Can you work these out from the model? Positions are in its coordinate system, mm. A direction names the side the tool comes from. Give positions to 0.01 mm unless a question says otherwise; leave off trailing zeros. Loops run counter-clockwise (first coordinate to the right, second up) from the corner with the lowest first, then second, coordinate; pieces in that order, holes last. Notation, with made-up numbers: (54, 58.25) - (94, 58.25) arc R29 cw to (94, 91.25) - close; hole circle Ø8 at (76, -27). An arc over 180 degrees is marked (long way). Write item = value, one per line.
from build123d import *

# Parameters (mm, degrees)
F0_R     = 6.75
F1_DEPTH = 8
F3_DEPTH = 8.001


with BuildPart() as f1:
    # F0 (on Right) → F1 (new body)
    with BuildSketch(Plane.YZ):
        Circle(F0_R)
    extrude(amount=F1_DEPTH)

    # F2 (on face) → F3 (cut, through all)
    with BuildSketch(Plane.YZ.offset(8)):
        with BuildLine():
            ThreePointArc((-1.426585, 0.463525), (-1.256585, 0.819143), (-0.999817, 1.118198))
            Line((-0.999817, 1.118198), (-3.928516, 3.849254))
            ThreePointArc((-3.928516, 3.849254), (-4.704102, 2.849811), (-5.230811, 1.699593))
            Line((-5.230811, 1.699593), (-1.426585, 0.463525))
        make_face()
        with BuildLine():
            Line((-3.232819, -4.449593), (-0.881678, -1.213525))
            ThreePointArc((-0.881678, -1.213525), (-1.167357, -0.941954), (-1.37243, -0.60534))
            Line((-1.37243, -0.60534), (-4.874837, -2.546756))
            ThreePointArc((-4.874837, -2.546756), (-4.163979, -3.593227), (-3.232819, -4.449593))
        make_face()
        with BuildLine():
            ThreePointArc((0, 1.5), (0.390745, 1.448212), (0.754509, 1.296424))
            Line((0.754509, 1.296424), (2.44688, 4.925726))
            ThreePointArc((2.44688, 4.925726), (1.256683, 5.354507), (0, 5.5))
            Line((0, 5.5), (0, 1.5))
        make_face()
        with BuildLine():
            Line((3.232819, -4.449593), (0.881678, -1.213525))
            ThreePointArc((0.881678, -1.213525), (0.535118, -1.401302), (0.151609, -1.492319))
            Line((0.151609, -1.492319), (0.915702, -5.423236))
            ThreePointArc((0.915702, -5.423236), (2.130622, -5.070547), (3.232819, -4.449593))
        make_face()
        with BuildLine():
            ThreePointArc((1.426585, 0.463525), (1.481533, 0.234652), (1.5, 0))
            ThreePointArc((1.5, 0), (1.491508, -0.159384), (1.466129, -0.316964))
            Line((1.466129, -0.316964), (5.440771, -0.804988))
            ThreePointArc((5.440771, -0.804988), (5.485173, -0.403582), (5.5, 0))
            ThreePointArc((5.5, 0), (5.432286, 0.86039), (5.230811, 1.699593))
            Line((5.230811, 1.699593), (1.426585, 0.463525))
        make_face()
    extrude(amount=-F3_DEPTH, mode=Mode.SUBTRACT)


solid = f1.part
Q1. Imagine slicing it at D-D, the plane y = 6.25. Write out the boundary of the cut face in (x, z).
Output:
outline = (0, -2.55) - (8, -2.55) - (8, 2.55) - (0, 2.55) - close
Q2. Which directions (+Z, -Z, +X, -X, +Y, -Y) give clear straight access to the entire face, cutting with the end or side of a thin tool? Please do faces 4 (the flat face through (8, 0, 0)), 5 (the flat face through (4.056, -3.099, -1.562)).
Output:
face_4 = +Z, -Z, +X, +Y, -Y
face_5 = +X, -X
Q3. For pin 1 (2 mm diameter, centred on x = 4, z = -4, fed in from +Y), with a flat end and sliding along its axis, tell me the tip position at first contact or that it passes through.
Output:
pin_1 = 6.05
Q4. We'd pull the mould along Y, two halves only. Please class faces 1 (the flat face through (4.06, -3.36, 1.09)), 2 (the flat face through (0, 0, 0)), 3 (the cylindrical face through (3.94, -1.46, -6.59)): released by +Y, released by -Y, zero draft, split by the parting line, or undercut.
Output:
face_1 = undercut
face_2 = zero draft
face_3 = split by the parting line
Q5. Imagine slicing it at B-B, the plane z = 2.75. Write out the boundary of the cut face in (x, y).
Output:
outline = (0, -6.16) - (8, -6.16) - (8, -4.76) - (0, -4.76) - close; (0, -2.75) - (8, -2.75) - (8, 0) - (0, 0) - close; (0, 1.43) - (8, 1.43) - (8, 6.16) - (0, 6.16) - close
Q6. Imagine slicing it at C-C, the plane y = 2. Write out the boundary of the cut face in (x, z).
Output:
outline = (0, -6.45) - (8, -6.45) - (8, -5.12) - (0, -5.12) - close; (0, -2.75) - (8, -2.75) - (8, -0.38) - (0, -0.38) - close; (0, 0.65) - (8, 0.65) - (8, 3.97) - (0, 3.97) - close; (0, 5.12) - (8, 5.12) - (8, 6.45) - (0, 6.45) - close
Q7. Imagine slicing it at A-A, the plane x = 3.5. Write out the boundary of the cut face in (y, z).
Output:
outline = circle Ø13.5 at (0, 0); hole (-5.23, 1.7) - (-1.43, 0.46) arc R1.5 cw to (-1, 1.12) - (-3.93, 3.85) arc R5.5 ccw to start; hole (-4.87, -2.55) arc R5.5 ccw to (-3.23, -4.45) - (-0.88, -1.21) arc R1.5 cw to (-1.37, -0.61) - close; hole (0, 1.5) arc R1.5 cw to (0.75, 1.3) - (2.45, 4.93) arc R5.5 ccw to (0, 5.5) - close; hole (0.15, -1.49) - (0.92, -5.42) arc R5.5 ccw to (3.23, -4.45) - (0.88, -1.21) arc R1.5 cw to start; hole (1.43, 0.46) arc R1.5 cw to (1.5, 0) arc R1.5 cw to (1.47, -0.32) - (5.44, -0.8) arc R5.5 ccw to (5.5, 0) arc R5.5 ccw to (5.23, 1.7) - close
Q8. I need wall thicknesses on L1, parallel to Z at x = 1.5, y = 1.75; L2, parallel to Y at x = 3.75, z = 3; L3, parallel to Z at x = 1.5, y = 2.5. Which ranges of each line are inside material? Lowest first, please.
Output:
L1 = -6.52 to -5.21, -2.41 to -0.35, 0.57 to 3.43, 5.21 to 6.52
L2 = -6.05 to -4.61, -3.02 to 0, 1.55 to 6.05
L3 = -6.27 to -4.9, -3.44 to -0.44, 0.81 to 6.27
